Geometry check sheet. Reference: the model listing, model coordinates, mm. A direction names the side the tool comes from. Round coordinates to 2 decimals unless told otherwise and drop trailing zeros. Write each loop counter-clockwise with the first axis right and the second up, starting at its lowest first coordinate (ties: lowest second). Pieces come first, ordered by that corner, then holes.
from build123d import *

# Parameters (mm, degrees)
SKETCH2_R           = 4
BOSS_EXTRUDE1_DEPTH = 0.2


with BuildPart() as part:
    # Sketch1 → Revolve1 (revolve)
    with BuildSketch(Plane.XY):
        Polygon((4, -3.313539221), (4, 9.698172784), (6.48, 9.698172784), (6.52, 14.698172784), (9.315596793, 14.698172784), (10.25, 10.692316782), (8.5, 3.192316782), (10.25, -4.307683218), (9.315596793, -8.313539221), (6.52, -8.313539221), (6.48, -3.313539221), align=None)
    revolve(axis=Axis((0, 42.323455848, 0), (0, -1, 0)))

    # Sketch2 → Boss-Extrude1 (add)
    with BuildSketch(Plane.XZ.offset(3.313539221)):
        Circle(SKETCH2_R)
    extrude(amount=-BOSS_EXTRUDE1_DEPTH)


solid = part.part
1. Depth check by flat-ended pin: pin 1 Ø1 at (y, z) = (7.5, -7) entering from -X; pin 2 Ø7 at (x, z) = (0, 0) entering from +Y; pin 3 Ø4 at (x, y) = (-3, 5.5) entering from -Z. Enter the tip coordinate at first touch or a pass-through.
2. Section check B-B (y = 7.75). Record the cut outline in (x, z), plus the area to 3 significant figures.
3. Release check for a two-part mould opening along X. For faces 5 (the face through (0, -3.114, 0)), 6 (the face through (-2.03, 14.45, -9.15)), 7 (the face through (3, 9.698, -3)), 8 (the face through (2.2, 14.698, 6.3)) record: +X half, -X half, draft (parallel to the pull), parting line (faces both ways), or undercut.
4. Section check A-A (y = -2.25). Record the cut outline in (x, z).
5. Scan lines: line 1 along Y through (x, z) = (-3.75, -4.5); line 2 along Z through (x, y) = (-1.75, -5.5); line 3 along Z through (x, y) = (0, 3). Record each from-to range of solid material in increasing order.
6. Access from +Z, -Z, +X, -X, +Y, -Y to the whole of each face (thin tool, end or side, straight path). Record for faces 1 (the face through (-1.409, 12.233, -6.346)), 2 (the face through (-2.2, -8.314, 6.3)), 3 (the face through (8.583, 1.056, 2.703)), 4 (the face through (0, -3.314, 0)).
Results below:
1. pin 1: stops at x = -6.96
1. pin 2: stops at y = -3.11
1. pin 3: stops at z = -9.24
2. outline: circle Ø19.13 at (0, 0); hole circle Ø8 at (0, 0)
2. area: 237 mm2
3. face 5: undercut
3. face 6: parting line
3. face 7: undercut
3. face 8: draft
4. outline: circle Ø19.54 at (0, 0); hole circle Ø8 at (0, 0)
5. line 1: y = -3.31 to 9.7
5. line 2: z = -9.82 to -6.26, 6.26 to 9.82
5. line 3: z = -8.54 to -4, 4 to 8.54
6. face 1: +Y
6. face 2: +Z, -Z, +X, -X, -Y
6. face 3: none
6. face 4: -Y
